The model under review builds one solid part; all positions refer to its coordinate system, in mm. A direction names the side the tool comes from. Coordinates: 2 decimals unless noted, no trailing zeros. Write each loop counter-clockwise with the first axis right and the second up, starting at its lowest first coordinate (ties: lowest second). Pieces come first, ordered by that corner, then holes. Notation, with made-up numbers: (42.25, 69.5) - (49.25, 69.5) arc R20 ccw to (49.25, 79.5) - close; hole circle Ø7 at (82.5, -32.75). An arc over 180 degrees is marked (long way). Put each result on its own line as item: value.
from build123d import *

# Parameters (mm, degrees)
CROQUIS1_R              = 7.5
SALIENTE_EXTRUIR1_DEPTH = 3
CROQUIS2_R              = 0.75
CROQUIS4_R              = 5
SALIENTE_EXTRUIR2_DEPTH = 29
CROQUIS5_R              = 6
SALIENTE_EXTRUIR3_DEPTH = 8
SALIENTE_EXTRUIR4_START = 3
CROQUIS6_R              = 5
SALIENTE_EXTRUIR4_DEPTH = 3
CROQUIS3_R              = 2.5
CORTAR_EXTRUIR1_DEPTH   = 45.288824776


with BuildPart() as part:
    # Croquis1 → Saliente-Extruir1 (new body)
    with BuildSketch(Plane(origin=(0, 0, 0), x_dir=(1, 0, 0), z_dir=(0, 1, 0))):
        with Locations(Location((0, 0, 0), (0, 0, 270))):
            Circle(CROQUIS1_R)
    extrude(amount=SALIENTE_EXTRUIR1_DEPTH)

    # Croquis2 → Cortar-Revolución1 (revolve, cut)
    with BuildSketch(Plane(origin=(0, 0, 0), x_dir=(0, 0, -1), z_dir=(1, 0, 0)), mode=Mode.PRIVATE) as cortar_revoluci_n1_sk:
        with Locations((7.5, 1.5)):
            Circle(CROQUIS2_R)
    revolve(cortar_revoluci_n1_sk.sketch.rotate(Axis((0, 3, 0), (0, -1, 0)), 180), axis=Axis((0, 3, 0), (0, -1, 0)), mode=Mode.SUBTRACT)

    # Croquis4 → Saliente-Extruir2 (add)
    with BuildSketch(Plane.XZ):
        with Locations(Location((0, 0, 0), (0, 0, 90))):
            Circle(CROQUIS4_R)
    extrude(amount=SALIENTE_EXTRUIR2_DEPTH)

    # Croquis5 → Saliente-Extruir3 (add)
    with BuildSketch(Plane(origin=(0, 3, 0), x_dir=(1, 0, 0), z_dir=(0, 1, 0))):
        with Locations(Location((0, 0, 0), (0, 0, 270))):
            Circle(CROQUIS5_R)
    extrude(amount=SALIENTE_EXTRUIR3_DEPTH)

    # Croquis6 → Saliente-Extruir4 (add)
    with BuildSketch(Plane(origin=(0, 11, 0), x_dir=(1, 0, 0), z_dir=(0, 1, 0)).offset(SALIENTE_EXTRUIR4_START)):
        with Locations(Location((0, 0, 0), (0, 0, 270))):
            Circle(CROQUIS6_R)
    extrude(amount=-SALIENTE_EXTRUIR4_DEPTH)

    # Croquis3 → Cortar-Extruir1 (cut, through all)
    with BuildSketch(Plane(origin=(0, -29, 0), x_dir=(1, 0, 0), z_dir=(0, 1, 0))):
        with Locations(Location((0, 0, 0), (0, 0, 270))):
            Circle(CROQUIS3_R)
    extrude(amount=CORTAR_EXTRUIR1_DEPTH, mode=Mode.SUBTRACT)


solid = part.part
1. To check wall thickness, follow probe 1 along X at (y, z) = (-10, 0); probe 2 along X at (y, z) = (5, 0); probe 3 along Y at (x, z) = (5, 1.25). State the ranges of each line that lie inside material, in increasing order.
Determined:
probe 1: x = -5 to -2.5, 2.5 to 5
probe 2: x = -6 to -2.5, 2.5 to 6
probe 3: y = 0 to 11
2. Consider section A-A on x = 0. State the section outline as (y, z) points.
Determined:
outline: (-29, -5) - (0, -5) - (0, -7.5) - (0.75, -7.5) arc R0.75 cw to (2.25, -7.5) - (3, -7.5) - (3, -6) - (11, -6) - (11, -5) - (14, -5) - (14, -2.5) - (-29, -2.5) - close; (-29, 2.5) - (14, 2.5) - (14, 5) - (11, 5) - (11, 6) - (3, 6) - (3, 7.5) - (2.25, 7.5) arc R0.75 cw to (0.75, 7.5) - (0, 7.5) - (0, 5) - (-29, 5) - close
3. For pin 1 Ø1.5 at (y, z) = (-11.5, 0.5) entering from +X; pin 2 Ø3 at (x, y) = (0.5, 6.5) entering from -Z; pin 3 Ø6 at (y, z) = (9, -6) entering from +X; pin 4 Ø6.5 at (x, z) = (0, 0) entering from -Y, all flat-tipped, find the tip position at first contact; note any pin that passes through.
Determined:
pin 1: stops at x = 5
pin 2: stops at z = -6
pin 3: stops at x = 5.2
pin 4: stops at y = -29
4. Machinability: for faces 1 (the cylindrical face through (0.33, 2.62, -7.493)), 2 (the cylindrical face through (4.88, -14.3, -1.08)), 3 (the cylindrical face through (1.802, 6.944, 5.723)), which of the approach directions +Z, -Z, +X, -X, +Y, -Y give a long, thin tool a straight path to every point of the face, cutting with its end or side? Answer none if there is none.
Determined:
face 1: +Y, -Y
face 2: -Y
face 3: +Y
5. Consider section B-B on z = 0. State the section outline as (x, y) points.
Determined:
outline: (-7.5, 0) - (-5, 0) - (-5, -29) - (-2.5, -29) - (-2.5, 14) - (-5, 14) - (-5, 11) - (-6, 11) - (-6, 3) - (-7.5, 3) - (-7.5, 2.25) arc R0.75 cw to (-7.5, 0.75) - close; (2.5, -29) - (5, -29) - (5, 0) - (7.5, 0) - (7.5, 0.75) arc R0.75 cw to (7.5, 2.25) - (7.5, 3) - (6, 3) - (6, 11) - (5, 11) - (5, 14) - (2.5, 14) - close
6. Consider section D-D on y = -5. State the section outline as (x, z) points.
Determined:
outline: circle Ø10 at (0, 0); hole circle Ø5 at (0, 0)
7. The part is to be moulded in two halves that separate along Z. For faces 4 (the cylindrical face through (-2.44, -7.8, -0.54)), 5 (the flat face through (6, 3, 2)), 6 (the cylindrical face through (0.33, 0.37, -7.493)), say which applies: +Z half, -Z half, draft (parallel to the pull), parting line (faces both ways), or undercut.
Determined:
face 4: undercut
face 5: draft
face 6: parting line
8. Consider section C-C on y = 8. State the section outline as (x, z) points, plus the area to 3 significant figures.
Determined:
outline: circle Ø12 at (0, 0); hole circle Ø5 at (0, 0)
area: 93.5 mm^2
